from build123d import *

# Parameters (mm, degrees)
SKETCH_1_R      = 2.4
EXTRUDE_1_DEPTH = 28
CHAMFER_1_SIZE  = 0.5
M3X0_51_D       = 2.5
M3X0_51_DEPTH   = 3
M3X0_51_TIP     = 0.751075774


with BuildPart() as part:
    # Эскиз1 → Бобышка-Вытянуть1 (new body)
    with BuildSketch(Plane(origin=(0, 0, 0), x_dir=(1, 0, 0), z_dir=(0, 1, 0))):
        with Locations(Location((0, 0, 0), (0, 0, 270))):
            Circle(SKETCH_1_R)
    extrude(amount=EXTRUDE_1_DEPTH)

    # Фаска1
    chamfer_1_edges = [part.edges().sort_by_distance(p)[0] for p in [
        (0, 28, -2.4),
    ]]
    chamfer(chamfer_1_edges, length=CHAMFER_1_SIZE)

    # Отверстие обработанное метчиком M3x0.51
    with Locations(Plane(origin=(0, 0, -2.4), x_dir=(-1, 0, 0), z_dir=(0, 0, -1))):
        with Locations((0, 9)):
            Hole(M3X0_51_D / 2, depth=M3X0_51_DEPTH)
            with Locations((0, 0, -(M3X0_51_DEPTH + M3X0_51_TIP / 2))):  # 118° drill point
                Cone(0, M3X0_51_D / 2, M3X0_51_TIP, mode=Mode.SUBTRACT)


solid = part.part
For this review, take the finished solid that the model builds, in its own axes (mm). Coordinates: 2 decimals unless noted, no trailing zeros. Loops run counter-clockwise (first coordinate to the right, second up) from the corner with the lowest first, then second, coordinate; pieces in that order, holes last. Notation, with made-up numbers: (39, 88) - (84, 88) arc R21 cw to (84, 119) - close; hole circle Ø2 at (3.25, 77). An arc over 180 degrees is marked (long way). Use a Markdown table: item, result. Add a question column.
Item 1: We need section A-A (z = 0). Give the boundary of the cut face in (x, y), and give its area (3 significant figures).
Item 2: We need section B-B (y = 2.75). Give the boundary of the cut face in (x, z), and give its area (3 significant figures).
Item 3: Mouldability with a two-part tool opening along Y and no side actions: class faces 1 (the face through (0, 28, 0)), 2 (the face through (2.024, 13.558, 1.29)), 3 (the face through (-0.16, 10.24, -0.88)), 4 (the face through (0, 0, 0)) as pulls with the +Y half, pulls with the -Y half, needs draft (parallel to the pull), parting line crosses it, or undercut.
Item 4: For line 1 (Y direction, x = 0, z = -0.4); line 2 (Z direction, x = -0.1, y = 6); line 3 (X direction, y = 9, z = -0.05), list the stretches that pass through material, from the lowest coordinate up.
Results list:
| question | item | result |
|---|---|---|
| 1 | outline | (-2.4, 0) - (2.4, 0) - (2.4, 27.5) - (1.9, 28) - (-1.9, 28) - (-2.4, 27.5) - close; hole circle Ø2.5 at (0, 9) |
| 1 | area | 129 mm^2 |
| 2 | outline | circle Ø4.8 at (0, 0) |
| 2 | area | 18.1 mm^2 |
| 3 | face 1 | pulls with the +Y half |
| 3 | face 2 | needs draft |
| 3 | face 3 | undercut |
| 3 | face 4 | pulls with the -Y half |
| 4 | line 1 | y = 0 to 7.75, 10.25 to 28 |
| 4 | line 2 | z = -2.4 to 2.4 |
| 4 | line 3 | x = -2.4 to -1.25, 1.25 to 2.4 |
